Input: part model. Units: mm. Frame: model coordinates. A direction names the side the tool comes from. Coordinates: 2 decimals unless noted, no trailing zeros. Order: outer loops, then holes, each group sorted by start corner. A loop starts at its lowest first (then second) coordinate and runs counter-clockwise, first axis right, second up. Notation, with made-up numbers: (29.25, -2.5) - (68.25, -2.5) arc R10 cw to (68.25, 13.5) - close; hole circle Ø10 at (-22.5, -0.75). An arc over 180 degrees is marked (long way). Use a Markdown table: item, result. Add a question column.
from build123d import *

# Parameters (mm, degrees)
F0_W     = 72.39
F0_H     = 72.39
F1_DEPTH = 12.7
F2_R     = 3.81
F3_DEPTH = 6.35
F5_DEPTH = 5.08
F7_DEPTH = 5.08
F8_W     = 4.1331201792
F8_H     = 7.04711047
F8_W_2   = 14.3668507226
F8_H_2   = 5.652282387
F9_DEPTH = 2.54


with BuildPart() as f1:
    # F0 (on Top) → F1 (new body)
    with BuildSketch(Plane.XY):
        with Locations((-36.195, -36.195)):
            Rectangle(F0_W, F0_H)
    extrude(amount=F1_DEPTH)

    # F2 (on face) → F3 (cut)
    with BuildSketch(Plane.XY.offset(12.7)):
        with Locations((-60.325, -12.065)):
            Circle(F2_R)
        with Locations((-61.5655786634, -36.195)):
            Circle(F2_R)
        with Locations((-61.5633073788, -60.325)):
            Circle(F2_R)
        with Locations((-36.195, -12.065)):
            Circle(F2_R)
        with Locations((-37.4355786634, -36.195)):
            Circle(F2_R)
        with Locations((-37.4333073788, -60.325)):
            Circle(F2_R)
        with Locations((-12.065, -12.065)):
            Circle(F2_R)
        with Locations((-13.3055786634, -36.195)):
            Circle(F2_R)
        with Locations((-13.3033073788, -60.325)):
            Circle(F2_R)
    extrude(amount=-F3_DEPTH, mode=Mode.SUBTRACT)

    # F4 (on face) → F5 (join)
    with BuildSketch(Plane(origin=(0, 0, 0), x_dir=(1, 0, 0), z_dir=(0, 0, -1))):
        Polygon((5.08, 42.545), (0, 42.545), (0, 29.845), (5.08, 29.845), (5.08, 19.685), (17.78, 19.685), (17.78, 52.705), (5.08, 52.705), align=None)
        Polygon((-29.845, -5.08), (-29.845, 0), (-42.545, 0), (-42.545, -5.08), (-52.705, -5.08), (-52.705, -17.78), (-19.685, -17.78), (-19.685, -5.08), align=None)
    extrude(amount=-F5_DEPTH)

    # F6 (on face) → F7 (cut)
    with BuildSketch(Plane(origin=(0, 0, 0), x_dir=(1, 0, 0), z_dir=(0, 0, -1))):
        Polygon((-44.1891504281, -29.484081471), (-56.8891504281, -29.484081471), (-56.8891504281, -42.184081471), (-44.1891504281, -42.184081471), (-44.1891504281, -54.884081471), (-31.4891504281, -54.884081471), (-31.4891504281, -17.78), (-44.1891504281, -17.78), align=None)
        Polygon((-72.39, 42.545), (-72.39, 29.845), (-67.31, 29.845), (-67.31, 19.685), (-54.61, 19.685), (-54.61, 52.705), (-67.31, 52.705), (-67.31, 42.545), align=None)
        Polygon((-29.845, 72.39), (-42.545, 72.39), (-42.545, 67.31), (-52.705, 67.31), (-52.705, 54.61), (-19.685, 54.61), (-19.685, 67.31), (-29.845, 67.31), align=None)
    extrude(amount=-F7_DEPTH, mode=Mode.SUBTRACT)

    # F8 (on face) → F9 (join)
    with BuildSketch(Plane(origin=(0, 0, 0), x_dir=(1, 0, 0), z_dir=(0, 0, -1))):
        with Locations((-36.4783331752, -0.2260982292)):
            Rectangle(F8_W, F8_H)
        with Locations((-3.0054978561, 35.1009014994)):
            Rectangle(F8_W_2, F8_H_2)
    extrude(amount=-F9_DEPTH)


solid = f1.part
1) Contact query for flat-ended pins moving along their axis: P1, Ø3, axis at x = -40.5, z = 9, coming from the +Y side; P2, Ø10, axis at x = -37.43, y = -60.32, coming from the -Z side; P3, Ø2.5, axis at y = 2, z = 3.5, coming from the +X side (3 decimals). Output: stop coordinate, or through.
2) Cut plane A-A (x = -26). Return the cut outline in (y, z).
3) Cut plane B-B (z = 10.75). State how many separate pieces and enclosed holes the cut face has, and give its area (3 significant figures).
4) Material intervals for L1, parallel to X at y = -29.5, z = 3.5; L2, parallel to X at y = -9.5, z = 8.25; L3, parallel to Y at x = -58, z = 1.75 (3 decimals), sorted ascending.
5) Reachability of faces 5 (the flat face through (-52.705, -61, 3)), 6 (the flat face through (5.08, -25, 3)), 7 (the cylindrical face through (-64.37, -57.75, 9.57)), 8 (the flat face through (-28, -27, 0)), 9 (the flat face through (-52.705, 11, 3)) from +Z, -Z, +X, -X, +Y, -Y: full face, straight path, thin tool, end or side. Return the list, or none.
6) Cut plane D-D (x = -7). Return the cut outline in (y, z), and give its area (3 significant figures).
7) Cut plane C-C (y = -38). Return the cut outline in (x, z), and give its area (3 significant figures).
8) Pull-direction query (X, two-part tool) for faces 1 (the flat face through (-37, -36, 6.35)), 2 (the flat face through (-72.39, -37, 6)), 3 (the flat face through (-25, 5.08, 3)), 4 (the flat face through (-62, -36, 5.08)); classes: pulls with the +X half, pulls with the -X half, needs draft (parallel to the pull), parting line crosses it, or undercut.
Computed:
| question | item | result |
|---|---|---|
| 1 | P1 | stops at y = 0 |
| 1 | P2 | stops at z = 5.08 |
| 1 | P3 | stops at x = -29.845 |
| 2 | outline | (-72.39, 0) - (-67.31, 0) - (-67.31, 5.08) - (-54.61, 5.08) - (-54.61, 0) - (0, 0) - (0, 12.7) - (-72.39, 12.7) - close; (5.08, 0) - (17.78, 0) - (17.78, 5.08) - (5.08, 5.08) - close |
| 3 | separate pieces | 1 |
| 3 | enclosed holes | 9 |
| 3 | area | 4,830 mm2 |
| 4 | L1 | x = -72.39 to -67.31, -54.61 to 0, 5.08 to 17.78 |
| 4 | L2 | x = -72.39 to -63.14, -57.51 to -39.01, -33.38 to -14.88, -9.25 to 0 |
| 4 | L3 | y = -72.39 to -52.705, -19.685 to 0 |
| 5 | face 5 | -Z |
| 5 | face 6 | +Z, -Z, +Y |
| 5 | face 7 | +Z |
| 5 | face 8 | -Z, +X, -X, +Y, -Y |
| 5 | face 9 | +Z, -Z, -X, +Y |
| 6 | outline | (-72.39, 0) - (0, 0) - (0, 12.7) - (-72.39, 12.7) - close |
| 6 | area | 919 mm2 |
| 7 | outline | (-72.39, 5.08) - (-54.61, 5.08) - (-54.61, 0) - (17.78, 0) - (17.78, 5.08) - (0, 5.08) - (0, 12.7) - (-9.95, 12.7) - (-9.95, 6.35) - (-16.66, 6.35) - (-16.66, 12.7) - (-34.08, 12.7) - (-34.08, 6.35) - (-40.79, 6.35) - (-40.79, 12.7) - (-58.21, 12.7) - (-58.21, 6.35) - (-64.92, 6.35) - (-64.92, 12.7) - (-72.39, 12.7) - close |
| 7 | area | 792 mm2 |
| 8 | face 1 | undercut |
| 8 | face 2 | pulls with the -X half |
| 8 | face 3 | needs draft |
| 8 | face 4 | undercut |
